The listing builds one solid part. Answer for the finished solid, in the listing's coordinates (mm). Face numbers are marked on the shaded views. A direction names the side the tool comes from. Coordinates: 2 decimals unless noted, no trailing zeros. Loops run counter-clockwise (first coordinate to the right, second up) from the corner with the lowest first, then second, coordinate; pieces in that order, holes last. Notation, with made-up numbers: (42, -10.5) - (72, -10.5) arc R18 ccw to (72, 16.5) - close; hole circle Ø3 at (34, 82.5). An arc over 180 degrees is marked (long way). Return JSON: item names as keys, results as strings. Group by question number.
1. Which of the six approach directions +Z, -Z, +X, -X, +Y, -Y give full straight-line access (tool end or side, diameter ignored) to the marked faces 1 and 2?
2. Section D-D (x = 39.5) is taken. Write down the section's boundary in (y, z).
3. Each of these flat-tipped pins is pushed along its axis until it touches: P1, Ø1.5, axis at y = -1, z = 44, coming from the -X side; P2, Ø3, axis at y = -8, z = 30.5, coming from the +X side; P3, Ø6, axis at x = -15.5, y = 4, coming from the +Z side. Where does it stop, or does it pass through?
4. Section A-A (y = -12) is taken. Write down the section's boundary in (x, z).
5. Section B-B (x = -7) is taken. Write down the section's boundary in (y, z).
6. Find the intervals of material crossed by line 1 along Z through (x, y) = (-28.5, 26.5); line 2 along X through (y, z) = (-12, 44.5); line 3 along Y through (x, z) = (-18.5, 37.5), in increasing order.
7. Section C-C (y = -36) is taken. Write down the section's boundary in (x, z).
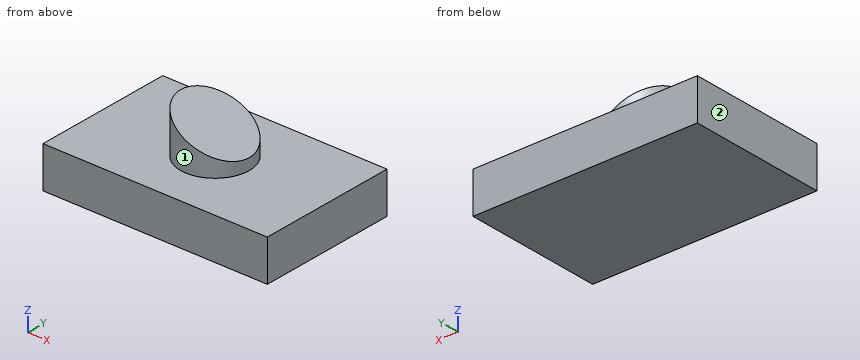
```python
from build123d import *

# Parameters (mm, degrees)
F0_W     = 136.481836
F0_H     = 85.016138
F0_R     = 20.850767
F1_DEPTH = 25
F2_DEPTH = 52.8
F4_DEPTH = 47.6


with BuildPart() as f1:
    # F0 (on Top) → F1 (new body)
    with BuildSketch(Plane.XY):
        Rectangle(F0_W, F0_H)
        Circle(F0_R, mode=Mode.SUBTRACT)
    extrude(amount=F1_DEPTH)

    # F0 (on Top) → F2 (join)
    with BuildSketch(Plane.XY):
        Circle(F0_R)
    extrude(amount=F2_DEPTH)

    # F3 (on Front) → F4 (cut, symmetric)
    with BuildSketch(Plane.XZ):
        Polygon((20.850767, 52.8), (-20.850767, 52.8), (20.850767, 31.842455), align=None)
    extrude(amount=F4_DEPTH, both=True, mode=Mode.SUBTRACT)


solid = f1.part
```
The answers:
{
 "1": {"face 1": "+Z", "face 2": "+Z, -Z, -X, +Y, -Y"},
 "2": {"outline": "(-42.51, 0) - (42.51, 0) - (42.51, 25) - (-42.51, 25) - close"},
 "3": {"P1": "stops at x = -20.85", "P2": "stops at x = 19.81", "P3": "stops at z = 51.62"},
 "4": {"outline": "(-68.24, 0) - (68.24, 0) - (68.24, 25) - (17.05, 25) - (17.05, 33.75) - (-17.05, 50.89) - (-17.05, 25) - (-68.24, 25) - close"},
 "5": {"outline": "(-42.51, 0) - (42.51, 0) - (42.51, 25) - (19.64, 25) - (19.64, 45.84) - (-19.64, 45.84) - (-19.64, 25) - (-42.51, 25) - close"},
 "6": {"line 1": "z = 0 to 25", "line 2": "x = -17.05 to -4.34", "line 3": "y = -9.62 to 9.62"},
 "7": {"outline": "(-68.24, 0) - (68.24, 0) - (68.24, 25) - (-68.24, 25) - close"}
}
